Geometry check sheet. Reference: drawing and pictorial views, mm from the part's lowest x, y, z. Coordinates: 2 decimals unless noted, no trailing zeros. Order: outer loops, then holes, each group sorted by start corner. A loop starts at its lowest first (then second) coordinate and runs counter-clockwise, first axis right, second up. Notation, with made-up numbers: M 19.5,89 L 67.5,89 A16 cw 67.5,111 Z; hole C 76,38 d1. An arc over 180 degrees is marked long. Return JSON: item names as keys, results as strings.
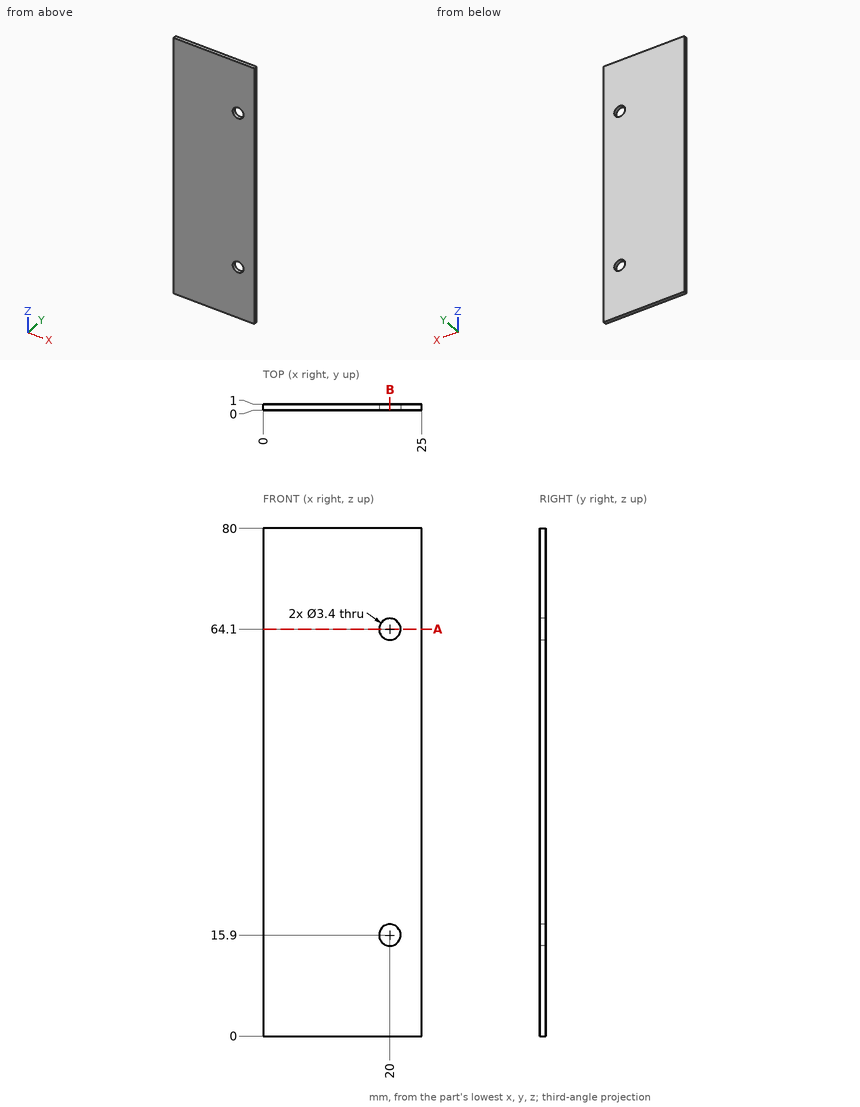
Q1. Material ranges on line 1 along Z through (x, y) = (20, 0.75); line 2 along X through (y, z) = (0.35, 64.1); line 3 along Z through (x, y) = (18.5, 0.9), recorded low to high.
Values:
{"line 1": "0 to 14.2, 17.6 to 62.4, 65.8 to 80", "line 2": "0 to 18.3, 21.7 to 25", "line 3": "0 to 15.1, 16.7 to 63.3, 64.9 to 80"}
Q2. Cross-section at A-A, the plane z = 64.1. Record the boundary of the cut face in (x, y), and give its area (3 significant figures).
Values:
{"outline": "M 0,0 L 18.3,0 L 18.3,1 L 0,1 Z; M 21.7,0 L 25,0 L 25,1 L 21.7,1 Z", "area": "21.6 mm^2"}
Q3. Cross-section at B-B, the plane x = 20. Record the boundary of the cut face in (y, z), and give its area (3 significant figures).
Values:
{"outline": "M 0,0 L 1,0 L 1,14.2 L 0,14.2 Z; M 0,17.6 L 1,17.6 L 1,62.4 L 0,62.4 Z; M 0,65.8 L 1,65.8 L 1,80 L 0,80 Z", "area": "73.2 mm^2"}
